```python
from build123d import *

# Parameters (mm, degrees)
SKETCH1_W             = 55
SKETCH1_H             = 30
BOSS_EXTRUDE1_DEPTH   = 12
SKETCH2_R             = 8.5
CUT_EXTRUDE1_DEPTH    = 34.544746235
SKETCH4_W             = 12
SKETCH4_H             = 5
CUT_EXTRUDE2_DEPTH    = 5
FILLET1_R             = 2
SKETCH5_W             = 12
SKETCH5_H             = 5
CUT_EXTRUDE3_DEPTH    = 3
FILLET2_R             = 5
BOSS_EXTRUDE3_DEPTH   = 8
F_3_0MM_DOWEL_HOLE1_D = 3


with BuildPart() as part:
    # Sketch1 → Boss-Extrude1 (new body)
    with BuildSketch(Plane(origin=(0, 0, 0), x_dir=(1, 0, 0), z_dir=(0, 1, 0))):
        Rectangle(SKETCH1_W, SKETCH1_H)
    extrude(amount=BOSS_EXTRUDE1_DEPTH)

    # Sketch2 → Cut-Extrude1 (cut, through all)
    with BuildSketch(Plane(origin=(0, 12, 0), x_dir=(1, 0, 0), z_dir=(0, 1, 0))):
        with Locations(Location((-13.12, 0, 0), (0, 0, 270))):
            Circle(SKETCH2_R)
        with Locations(Location((13.12, 0, 0), (0, 0, 270))):
            Circle(SKETCH2_R)
    extrude(amount=-CUT_EXTRUDE1_DEPTH, mode=Mode.SUBTRACT)

    # Sketch4 → Cut-Extrude2 (cut)
    with BuildSketch(Plane.XZ):
        with Locations((0, -10)):
            Rectangle(SKETCH4_W, SKETCH4_H)
    extrude(amount=-CUT_EXTRUDE2_DEPTH, mode=Mode.SUBTRACT)

    # Fillet1
    fillet1_edges = [part.edges().sort_by_distance(p)[0] for p in [
        (-6, 2.5, -12.5),
        (-6, 2.5, -7.5),
        (6, 2.5, -7.5),
        (6, 2.5, -12.5),
    ]]
    fillet(fillet1_edges, radius=FILLET1_R)

    # Sketch5 → Cut-Extrude3 (cut)
    with BuildSketch(Plane.XZ):
        with Locations((0, 12.5)):
            Rectangle(SKETCH5_W, SKETCH5_H)
    extrude(amount=-CUT_EXTRUDE3_DEPTH, mode=Mode.SUBTRACT)

    # Fillet2
    fillet2_edges = [part.edges().sort_by_distance(p)[0] for p in [
        (27.5, 6, 15),
        (-27.5, 6, 15),
        (-27.5, 6, -15),
        (27.5, 6, -15),
    ]]
    fillet(fillet2_edges, radius=FILLET2_R)

    # Sketch6 → Boss-Extrude3 (add)
    with BuildSketch(Plane.XZ):
        with BuildLine():
            Line((25.5, 10), (25.5, -10))
            ThreePointArc((25.5, -10), (24.621320344, -12.121320344), (22.5, -13))
            Line((22.5, -13), (-22.5, -13))
            ThreePointArc((-22.5, -13), (-24.621320344, -12.121320344), (-25.5, -10))
            Line((-25.5, -10), (-25.5, 10))
            ThreePointArc((-25.5, 10), (-24.621320344, 12.121320344), (-22.5, 13))
            Line((-22.5, 13), (-8, 13))
            Line((-8, 13), (-6, 13))
            Line((-6, 13), (-6, 15))
            Line((-6, 15), (-22.5, 15))
            ThreePointArc((-22.5, 15), (-26.035533906, 13.535533906), (-27.5, 10))
            Line((-27.5, 10), (-27.5, -10))
            ThreePointArc((-27.5, -10), (-26.035533906, -13.535533906), (-22.5, -15))
            Line((-22.5, -15), (22.5, -15))
            ThreePointArc((22.5, -15), (26.035533906, -13.535533906), (27.5, -10))
            Line((27.5, -10), (27.5, 10))
            ThreePointArc((27.5, 10), (26.035533906, 13.535533906), (22.5, 15))
            Line((22.5, 15), (6, 15))
            Line((6, 15), (6, 13))
            Line((6, 13), (8, 13))
            Line((8, 13), (22.5, 13))
            ThreePointArc((22.5, 13), (24.621320344, 12.121320344), (25.5, 10))
        make_face()
    extrude(amount=BOSS_EXTRUDE3_DEPTH)

    # Ø3.0mm Dowel Hole1 (through all)
    with Locations(Plane.ZY.offset(27.5)):
        with Locations((0, -5)):
            Hole(F_3_0MM_DOWEL_HOLE1_D / 2)


solid = part.part
```
The listing builds one solid part. Answer for the finished solid, in the listing's coordinates (mm). A direction names the side the tool comes from. Give positions to 0.01 mm unless a question says otherwise; leave off trailing zeros. Write each loop counter-clockwise with the first axis right and the second up, starting at its lowest first coordinate (ties: lowest second). Pieces come first, ordered by that corner, then holes. Notation, with made-up numbers: (81.5, 14.25) -> (125.5, 14.25) arc R22 cw to (125.5, 45.25) -> close; hole circle Ø2 at (54, -10). An arc over 180 degrees is marked (long way). Write item = value, one per line. Start each with the question number.
1) Determine the mould class of faces 4 (the face through (-6, 2, -10)), 5 (the face through (0, 12, 0)), 6 (the face through (0, 1, 10)) for opening direction Z: +Z half, -Z half, draft (parallel to the pull), parting line (faces both ways), or undercut.
2) Straight lines are drawn through the part: line 1 along X through (y, z) = (8.25, 0); line 2 along X through (y, z) = (1.75, -6.5); line 3 along Z through (x, y) = (13, -3.25). For each, find the intervals that lie inside material, in ascending order.
3) The part is cut by section A-A, the plane z = 0. Determine the outline of the cut face in (x, y).
4) The part is cut by section B-B, the plane x = -13.12. Determine the outline of the cut face in (y, z), and give its area (3 significant figures).
5) The part is cut by section C-C, the plane y = 7. Determine the outline of the cut face in (x, z).
6) Which of the six approach directions +Z, -Z, +X, -X, +Y, -Y give full straight-line access (tool end or side, diameter ignored) to faces 1 (the face through (0, 3, 13)), 2 (the face through (27.5, 2, 0)), 3 (the face through (0, 2, -12.5))?
7) The part is cut by section D-D, the plane y = -5. Determine the outline of the cut face in (x, z), and give its area (3 significant figures).
8) Each of these flat-tipped pins is pushed along its axis until it touches: pin 1 (4 mm diameter, centred on x = -2.5, z = 3.5, fed in from -Y); pin 2 (1.5 mm diameter, centred on x = 3.5, y = -1.5, fed in from +Z); pin 3 (2.5 mm diameter, centred on x = 2.5, z = 12.5, fed in from -Y). Where does it stop, or does it pass through?
Solutions:
q1.face_4 = undercut
q1.face_5 = draft
q1.face_6 = +Z half
q2.line_1 = -27.5 to -21.62, -4.62 to 4.62, 21.62 to 27.5
q2.line_2 = -27.5 to -18.6, -7.64 to 7.64, 18.6 to 27.5
q2.line_3 = -15 to -13, 13 to 15
q3.outline = (-27.5, -8) -> (-25.5, -8) -> (-25.5, -6.5) -> (-27.5, -6.5) -> close; (-27.5, -3.5) -> (-25.5, -3.5) -> (-25.5, 0) -> (-21.62, 0) -> (-21.62, 12) -> (-27.5, 12) -> close; (-4.62, 0) -> (4.62, 0) -> (4.62, 12) -> (-4.62, 12) -> close; (21.62, 0) -> (25.5, 0) -> (25.5, -3.5) -> (27.5, -3.5) -> (27.5, 12) -> (21.62, 12) -> close; (25.5, -8) -> (27.5, -8) -> (27.5, -6.5) -> (25.5, -6.5) -> close
q4.outline = (-8, -15) -> (12, -15) -> (12, -8.5) -> (0, -8.5) -> (0, -13) -> (-8, -13) -> close; (-8, 13) -> (0, 13) -> (0, 8.5) -> (12, 8.5) -> (12, 15) -> (-8, 15) -> close
q4.area = 188 mm²
q5.outline = (-27.5, -10) arc R5 ccw to (-22.5, -15) -> (22.5, -15) arc R5 ccw to (27.5, -10) -> (27.5, 10) arc R5 ccw to (22.5, 15) -> (-22.5, 15) arc R5 ccw to (-27.5, 10) -> close; hole circle Ø17 at (-13.12, 0); hole circle Ø17 at (13.12, 0)
q6.face_1 = +Z, -Y
q6.face_2 = +Z, -Z, +X, +Y, -Y
q6.face_3 = -Y
q7.outline = (-27.5, -10) arc R5 ccw to (-22.5, -15) -> (22.5, -15) arc R5 ccw to (27.5, -10) -> (27.5, -1.5) -> (25.5, -1.5) -> (25.5, -10) arc R3 cw to (22.5, -13) -> (-22.5, -13) arc R3 cw to (-25.5, -10) -> (-25.5, -1.5) -> (-27.5, -1.5) -> close; (-27.5, 1.5) -> (-25.5, 1.5) -> (-25.5, 10) arc R3 cw to (-22.5, 13) -> (-6, 13) -> (-6, 15) -> (-22.5, 15) arc R5 ccw to (-27.5, 10) -> close; (6, 13) -> (22.5, 13) arc R3 cw to (25.5, 10) -> (25.5, 1.5) -> (27.5, 1.5) -> (27.5, 10) arc R5 ccw to (22.5, 15) -> (6, 15) -> close
q7.area = 274 mm²
q8.pin_1 = 0
q8.pin_2 = -13
q8.pin_3 = 3
